Check sheet for the modelled part. Datum: model origin and axes. Units: mm. A direction names the side the tool comes from. Coordinates: 2 decimals unless noted, no trailing zeros. Order: outer loops, then holes, each group sorted by start corner. A loop starts at its lowest first (then second) coordinate and runs counter-clockwise, first axis right, second up.
1. Cross-section at A-A (x = 10.5). Enter the section's corners in (y, z).
2. Gauge pin test, flat ends, axial feed: pin 1 Ø1 at (y, z) = (6.5, 5.5) entering from +X; pin 2 Ø3 at (x, z) = (13, 5) entering from +Y; pin 3 Ø3 at (x, y) = (11, 2) entering from -Z; pin 4 Ø3.5 at (x, z) = (15, 10) entering from +Y. Record the tip position at first contact, or that the pin passes through.
3. Set-up check for faces 4 (the flat face through (2, 11, 12.75)), 5 (the flat face through (2, 19.2, 10)), 6 (the flat face through (11, 2, 7.25)), 7 (the flat face through (8, 8, 4.5)), 8 (the flat face through (8, 8, 20)): record each of +Z, -Z, +X, -X, +Y, -Y from which the full face is reachable in a straight line by a thin tool's end or side.
4. Cross-section at C-C (z = 17). Enter the section's corners in (x, y), then the cut area to 3 significant figures.
5. Cross-section at B-B (y = 11.5). Enter the section's corners in (x, z).
6. Draft check along Z on faces 1 (the flat face through (2, 11, 7.25)), 2 (the flat face through (8, 8, 0)), 3 (the flat face through (0, 7.6, 12.1)). Enter one of: released by +Z, released by -Z, zero draft, split by the parting line, or undercut.
7. Thickness scan on line 1 (Z direction, x = 12.25, y = 9); line 2 (X direction, y = 10.75, z = 13.75); line 3 (Z direction, x = 3, y = 13). Record the ranges inside material, lowest first.
8. Cross-section at D-D (y = 17). Enter the section's corners in (x, z), then the cut area to 3 significant figures.
```python
from build123d import *

# Parameters (mm, degrees)
BOSS_EXTRUDE1_DEPTH = 4.5
BOSS_EXTRUDE2_DEPTH = 4


with BuildPart() as part:
    # Sketch1 → Boss-Extrude1 (new body)
    with BuildSketch(Plane.XY):
        Polygon((0, 0), (0, 19.2), (4, 19.2), (11.6, 11.6), align=None)
    extrude(amount=BOSS_EXTRUDE1_DEPTH)

    # Sketch2 → Boss-Extrude2 (add)
    with BuildSketch(Plane(origin=(0, 0, 0), x_dir=(0, 0, -1), z_dir=(1, 0, 0))):
        with BuildLine():
            Line((-4.5, 19.2), (-10, 19.2))
            Line((-10, 19.2), (-10, 15.7))
            ThreePointArc((-10, 15.7), (-8.055456352, 14.894543648), (-7.25, 12.95))
            Line((-7.25, 12.95), (-7.25, 10))
            ThreePointArc((-7.25, 10), (-8.055456352, 8.055456352), (-10, 7.25))
            Line((-10, 7.25), (-10, 0))
            Line((-10, 0), (-4.5, 0))
            Line((-4.5, 0), (-4.5, 19.2))
        make_face()
    extrude(amount=BOSS_EXTRUDE2_DEPTH)

    # Mirror3: part across plane


with BuildPart() as part_1:
    add(part.part)
    add(part.part.mirror(Plane(origin=(4, 19.2, 10), x_dir=(1, 0, 0), z_dir=(0, 0, -1))))

    # Mirror4: part across plane


with BuildPart() as part_2:
    add(part_1.part)
    add(part_1.part.mirror(Plane(origin=(0, 0, 15.5), x_dir=(0, 0, 1), z_dir=(-0.7071067811865475, 0.7071067811865477, 0))))


solid = part_2.part
```
Data:
1. outline: (0, 0) - (12.7, 0) - (12.7, 4.5) - (4, 4.5) - (4, 7.25) - (0, 7.25) - close; (0, 12.75) - (4, 12.75) - (4, 15.5) - (12.7, 15.5) - (12.7, 20) - (0, 20) - close
2. pin 1: stops at x = 4
2. pin 2: stops at y = 11.61
2. pin 3: stops at z = 0
2. pin 4: stops at y = 4
3. face 4: +X, -X
3. face 5: +Z, -Z, +X, -X, +Y
3. face 6: +Y, -Y
3. face 7: +X, +Y
3. face 8: +Z, +X, -X, +Y, -Y
4. outline: (0, 0) - (19.2, 0) - (19.2, 4) - (4, 19.2) - (0, 19.2) - close
4. area: 253 mm2
5. outline: (0, 0) - (11.7, 0) - (11.7, 4.5) - (4, 4.5) - (4, 7.25) - (0, 7.25) - close; (0, 12.75) - (4, 12.75) - (4, 15.5) - (11.7, 15.5) - (11.7, 20) - (0, 20) - close
6. face 1: undercut
6. face 2: released by -Z
6. face 3: zero draft
7. line 1: z = 0 to 4.5, 15.5 to 20
7. line 2: x = 0 to 4
7. line 3: z = 0 to 7.25, 12.75 to 20
8. outline: (0, 0) - (6.2, 0) - (6.2, 4.5) - (4, 4.5) - (4, 15.5) - (6.2, 15.5) - (6.2, 20) - (0, 20) - close
8. area: 99.8 mm2
